```python
from build123d import *

# Parameters (mm, degrees)
BOSS_EXTRUDE1_DEPTH = 25.4
SKETCH2_R           = 25.4
BOSS_EXTRUDE2_DEPTH = 12.7


with BuildPart() as part:
    # Sketch1 → Boss-Extrude1 (new body, symmetric)
    with BuildSketch(Plane.XY):
        Polygon((-38.1, 0), (38.1, 0), (50.8, 26.773950856), (50.8, 76.2), (38.1, 76.2), (38.1, 44.45), (25.4, 17.676049144), (-25.4, 17.676049144), (-38.1, 44.45), (-38.1, 76.2), (-50.8, 76.2), (-50.8, 26.773950856), align=None)
    extrude(amount=BOSS_EXTRUDE1_DEPTH, both=True)

    # Sketch2 → Boss-Extrude2 (add)
    with BuildSketch(Plane.XZ):
        Circle(SKETCH2_R)
    extrude(amount=BOSS_EXTRUDE2_DEPTH)


solid = part.part
```
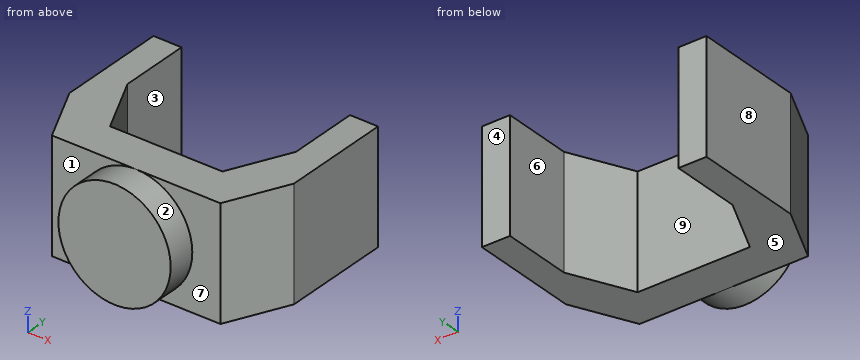
Verification items for the finished model (mm, model axes). Face numbers are marked on the shaded views. A direction names the side the tool comes from. Give positions to 0.01 mm unless a question says otherwise; leave off trailing zeros. Write each loop counter-clockwise with the first axis right and the second up, starting at its lowest first coordinate (ties: lowest second). Pieces come first, ordered by that corner, then holes. Notation, with made-up numbers: (-7, 14) - (32, 14) arc R20 cw to (32, 25) - close; hole circle Ø8 at (34.25, -39.5). An arc over 180 degrees is marked (long way). Put each result on its own line as item: value.
Q1. Scan lines: probe 1 along X at (y, z) = (68, 0.5); probe 2 along Y at (x, z) = (15, -8.5); probe 3 along X at (y, z) = (19, -7.5). Record each from-to range of solid material in increasing order. Write a range as from..to.
Result:
probe 1: -50.8..-38.1, 38.1..50.8
probe 2: -12.7..17.68
probe 3: -47.11..-26.03, 26.03..47.11
Q2. Section check C-C on x = 6. Record the cut outline in (y, z), and give its area (3 significant figures).
Result:
outline: (-12.7, -24.68) - (0, -24.68) - (0, -25.4) - (17.68, -25.4) - (17.68, 25.4) - (0, 25.4) - (0, 24.68) - (-12.7, 24.68) - close
area: 1,520 mm2
Q3. Section check D-D on y = 42. Record the cut outline in (x, z), and give its area (3 significant figures).
Result:
outline: (-50.8, -25.4) - (-36.94, -25.4) - (-36.94, 25.4) - (-50.8, 25.4) - close; (36.94, -25.4) - (50.8, -25.4) - (50.8, 25.4) - (36.94, 25.4) - close
area: 1,410 mm2
Q4. Depth check by flat-ended pin: P1, Ø15, axis at x = 3.5, z = -0.5, coming from the +Y side; P2, Ø12, axis at x = 28, y = 26.5, coming from the -Z side. Enter the tip coordinate at first touch or a pass-through.
Result:
P1: y = 17.68
P2: z = -25.4
Q5. Set-up check for the marked faces 1, 2, 3, 4 and 5: record each of +Z, -Z, +X, -X, +Y, -Y from which the full face is reachable in a straight line by a thin tool's end or side.
Result:
face 1: -X, -Y
face 2: -Y
face 3: +Z, -Z, +Y
face 4: +Z, -Z, +X, -X, +Y
face 5: -Z, +X, -X, +Y, -Y
Q6. Section check B-B on z = 0. Record the cut outline in (x, y).
Result:
outline: (-50.8, 26.77) - (-38.1, 0) - (-25.4, 0) - (-25.4, -12.7) - (25.4, -12.7) - (25.4, 0) - (38.1, 0) - (50.8, 26.77) - (50.8, 76.2) - (38.1, 76.2) - (38.1, 44.45) - (25.4, 17.68) - (-25.4, 17.68) - (-38.1, 44.45) - (-38.1, 76.2) - (-50.8, 76.2) - close
Q7. Mould release check, pull along X, two halves, no side actions. Record for the marked faces 6, 7, 8 and 9: released by +X, released by -X, zero draft, split by the parting line, or undercut.
Result:
face 6: undercut
face 7: zero draft
face 8: released by -X
face 9: undercut
Q8. Section check A-A on y = 52. Record the cut outline in (x, z).
Result:
outline: (-50.8, -25.4) - (-38.1, -25.4) - (-38.1, 25.4) - (-50.8, 25.4) - close; (38.1, -25.4) - (50.8, -25.4) - (50.8, 25.4) - (38.1, 25.4) - close
